from build123d import *

# Parameters (mm, degrees)
BOSS_EXTRUDE1_DEPTH = 3
SKETCH3_R           = 2
CUT_EXTRUDE5_DEPTH  = 10
SKETCH4_R           = 4
CUT_EXTRUDE6_DEPTH  = 10
SKETCH6_R           = 2
CUT_EXTRUDE7_DEPTH  = 10
SKETCH8_R           = 2.5
CUT_EXTRUDE8_DEPTH  = 55


with BuildPart() as part:
    # Sketch2 → Boss-Extrude1 (new body)
    with BuildSketch(Plane(origin=(0, 0, 0), x_dir=(1, 0, 0), z_dir=(0, 1, 0))):
        with BuildLine():
            Line((2.81621534, -115.073455489), (52.81621534, -115.073455489))
            Line((52.81621534, -115.073455489), (52.81621534, -315.073455489))
            Line((52.81621534, -315.073455489), (2.81621534, -315.073455489))
            Line((2.81621534, -315.073455489), (2.81621534, -382.433365135))
            ThreePointArc((2.81621534, -382.433365135), (202.81621534, -465.073455489), (402.81621534, -382.433365135))
            Line((402.81621534, -382.433365135), (402.81621534, -315.073455489))
            Line((402.81621534, -315.073455489), (352.81621534, -315.073455489))
            Line((352.81621534, -315.073455489), (352.81621534, -115.073455489))
            Line((352.81621534, -115.073455489), (402.81621534, -115.073455489))
            Line((402.81621534, -115.073455489), (402.81621534, -47.713545842))
            ThreePointArc((402.81621534, -47.713545842), (202.81621534, 34.926544511), (2.81621534, -47.713545842))
            Line((2.81621534, -47.713545842), (2.81621534, -115.073455489))
        make_face()
    extrude(amount=BOSS_EXTRUDE1_DEPTH)

    # Sketch3 → Cut-Extrude5 (cut)
    with BuildSketch(Plane(origin=(0, 3, 0), x_dir=(1, 0, 0), z_dir=(0, 1, 0))):
        with Locations(Location((64.81621534, -196.073455489, 0), (0, 0, 270))):
            Circle(SKETCH3_R)
        with Locations(Location((104.81621534, -196.073455489, 0), (0, 0, 270))):
            Circle(SKETCH3_R)
        with Locations(Location((104.81621534, -234.073455489, 0), (0, 0, 90))):
            Circle(SKETCH3_R)
        with Locations(Location((64.81621534, -234.073455489, 0), (0, 0, 90))):
            Circle(SKETCH3_R)
        with Locations(Location((340.81621534, -234.073455489, 0), (0, 0, 270))):
            Circle(SKETCH3_R)
        with Locations(Location((300.81621534, -234.073455489, 0), (0, 0, 270))):
            Circle(SKETCH3_R)
        with Locations(Location((300.81621534, -196.073455489, 0), (0, 0, 90))):
            Circle(SKETCH3_R)
        with Locations(Location((340.81621534, -196.073455489, 0), (0, 0, 90))):
            Circle(SKETCH3_R)
    extrude(amount=-CUT_EXTRUDE5_DEPTH, mode=Mode.SUBTRACT)

    # Sketch4 → Cut-Extrude6 (cut)
    with BuildSketch(Plane(origin=(0, 3, 0), x_dir=(1, 0, 0), z_dir=(0, 1, 0))):
        with Locations(Location((52.81621534, -47.713545842, 0), (0, 0, 270))):
            Circle(SKETCH4_R)
        with Locations(Location((352.81621534, -47.713545842, 0), (0, 0, 90))):
            Circle(SKETCH4_R)
        with Locations(Location((352.81621534, -382.433365135, 0), (0, 0, 270))):
            Circle(SKETCH4_R)
        with Locations(Location((52.81621534, -382.433365135, 0), (0, 0, 90))):
            Circle(SKETCH4_R)
    extrude(amount=-CUT_EXTRUDE6_DEPTH, mode=Mode.SUBTRACT)

    # Sketch6 → Cut-Extrude7 (cut)
    with BuildSketch(Plane(origin=(0, 3, 0), x_dir=(1, 0, 0), z_dir=(0, 1, 0))):
        with Locations(Location((139.31621534, -263.573455489, 0), (0, 0, 270))):
            Circle(SKETCH6_R)
        with Locations(Location((139.31621534, -166.573455489, 0), (0, 0, 270))):
            Circle(SKETCH6_R)
        with Locations(Location((266.31621534, -166.573455489, 0), (0, 0, 270))):
            Circle(SKETCH6_R)
        with Locations(Location((266.31621534, -263.573455489, 0), (0, 0, 270))):
            Circle(SKETCH6_R)
    extrude(amount=-CUT_EXTRUDE7_DEPTH, mode=Mode.SUBTRACT)

    # Sketch8 → Cut-Extrude8 (cut)
    with BuildSketch(Plane(origin=(0, 3, 0), x_dir=(1, 0, 0), z_dir=(0, 1, 0))):
        with Locations(Location((168.25621534, -333.473365135, 0), (0, 0, 270))):
            Circle(SKETCH8_R)
        with Locations(Location((237.37621534, -333.473365135, 0), (0, 0, 270))):
            Circle(SKETCH8_R)
        with Locations(Location((237.37621534, -431.393365135, 0), (0, 0, 270))):
            Circle(SKETCH8_R)
        with Locations(Location((168.25621534, -431.393365135, 0), (0, 0, 270))):
            Circle(SKETCH8_R)
        with Locations(Location((168.25621534, 1.246454158, 0), (0, 0, 90))):
            Circle(SKETCH8_R)
        with Locations(Location((237.37621534, 1.246454158, 0), (0, 0, 90))):
            Circle(SKETCH8_R)
        with Locations(Location((237.37621534, -96.673545842, 0), (0, 0, 90))):
            Circle(SKETCH8_R)
        with Locations(Location((168.25621534, -96.673545842, 0), (0, 0, 90))):
            Circle(SKETCH8_R)
    extrude(amount=-CUT_EXTRUDE8_DEPTH, mode=Mode.SUBTRACT)


solid = part.part
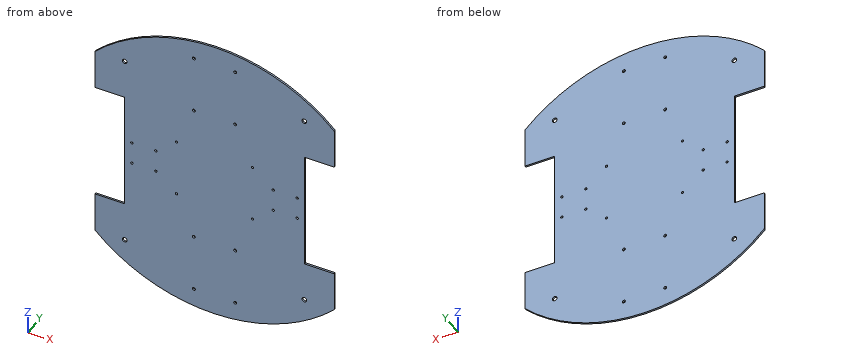
The listing builds one solid part. Answer for the finished solid, in the listing's coordinates (mm). Give positions to 0.01 mm unless a question says otherwise; leave off trailing zeros. Write each loop counter-clockwise with the first axis right and the second up, starting at its lowest first coordinate (ties: lowest second). Pieces come first, ordered by that corner, then holes. Notation, with made-up numbers: (32, -27.75) -> (57, -27.75) arc R11 ccw to (57, -16.75) -> close; hole circle Ø11 at (6.5, 3.25). An arc over 180 degrees is marked (long way). Use a Markdown table: item, result.
(1) Section B-B, the plane y = 2.4 is taken. Give the number of separate pieces and of enclosed holes in the cut face, then the cut area to 3 significant figures.
Return value:
| item | result |
|---|---|
| separate pieces | 1 |
| enclosed holes | 24 |
| area | 159,000 mm2 |
(2) Section A-A, the plane z = 158 is taken. Determine the outline of the cut face in (x, y).
Return value:
| item | result |
|---|---|
| outline | (52.82, 0) -> (352.82, 0) -> (352.82, 3) -> (52.82, 3) -> close |
(3) Find the intervals of material crossed by probe 1 along X at (y, z) = (1.45, 334); probe 2 along X at (y, z) = (2.6, 98); probe 3 along X at (y, z) = (1.95, 182), in increasing order. Write a range as from..to.
Return value:
| item | result |
|---|---|
| probe 1 | 2.82..165.81, 170.7..234.93, 239.82..402.82 |
| probe 2 | 2.82..166.14, 170.38..235.26, 239.5..402.82 |
| probe 3 | 52.82..352.82 |
(4) Section C-C, the plane x = 156.5 is taken. Determine the outline of the cut face in (y, z).
Return value:
| item | result |
|---|---|
| outline | (0, -31.12) -> (3, -31.12) -> (3, 461.26) -> (0, 461.26) -> close |
(5) Flat-ended cylindrical pins translate along their axes: P1, Ø1.5, axis at x = 17.5, y = 2, coming from the +Z side; P2, Ø0.9, axis at x = 375, y = 1, coming from the +Z side; P3, Ø0.9, axis at y = 1, z = 184, coming from the +X side. Find the tip coordinate at first contact, or state that the pin passes through.
Return value:
| item | result |
|---|---|
| P1 | z = 396.71 |
| P2 | z = 407.1 |
| P3 | x = 352.82 |
